Could you check a few things on this model? Use its own coordinates, in mm. A direction names the side the tool comes from. Coordinates: 2 decimals unless noted, no trailing zeros. Order: outer loops, then holes, each group sorted by start corner. A loop starts at its lowest first (then second) coordinate and runs counter-clockwise, first axis right, second up. Notation, with made-up numbers: (14, 76.5) -> (70, 76.5) arc R6 cw to (70, 80.5) -> close; hole circle Ø7 at (42.25, 82.25). An arc over 180 degrees is marked (long way). Put each result on its own line as item: value. Start each with the question number.
Q1. If we section it at C-C (z = 26): Please give me the cut outline in (x, y), and give its area (3 significant figures).
Q2. If we section it at B-B (y = -20): Please give me the cut outline in (x, z).
Q3. If we section it at D-D (y = -49): Please give me the cut outline in (x, z), and give its area (3 significant figures).
Q4. Please list where these lines run through material, in increasing order: line 1 along X through (y, z) = (-22.5, 0.75); line 2 along X through (y, z) = (-49, 41); line 3 along X through (y, z) = (-97, 1).
Q5. For faces 4 (the face through (24.73, -101.27, 1.38)), 5 (the face through (54.59, -59.16, 3.64)), which set-ups out of +Z, -Z, +X, -X, +Y, -Y let a thin tool reach every point of the face, with its end or its side?
Q6. We'd pull the mould along X, two halves only. Please class faces 1 (the face through (-46.17, -59.16, 3.6)), 2 (the face through (-48.21, -59.16, 1.68)), 3 (the face through (56.811, -12.675, 32.28)): +X half, -X half, draft (parallel to the pull), parting line (faces both ways), or undercut.
Q7. Will these pins go through, and if not, where does the flat tip stop? pin 1 (7 mm diameter, centred on x = -18.31, y = -22.5, fed in from +Z); pin 2 (4 mm diameter, centred on x = -4, y = -34.5, fed in from -Z); pin 3 (10 mm diameter, centred on x = 26.69, y = -22.5, fed in from +Z).
Q8. If we section it at A-A (z = 18): Please give me the cut outline in (x, y), and give its area (3 significant figures).
from build123d import *

# Parameters (mm, degrees)
F1_DEPTH = 120
F3_DEPTH = 3
F4_R     = 4.25
F5_DEPTH = 3


with BuildPart() as f1:
    # F0 (on Front) → F1 (new body)
    with BuildSketch(Plane.XZ):
        with BuildLine():
            ThreePointArc((-49.808191, 5.6), (-48.167989, 1.640202), (-44.208191, 0))
            Line((-44.208191, 0), (52.591809, 0))
            ThreePointArc((52.591809, 0), (56.551607, 1.640202), (58.191809, 5.6))
            Line((58.191809, 5.6), (58.191809, 52))
            Line((58.191809, 52), (55.391809, 52))
            Line((55.391809, 52), (55.391809, 5.6))
            ThreePointArc((55.391809, 5.6), (54.571708, 3.620101), (52.591809, 2.8))
            Line((52.591809, 2.8), (6.991809, 2.8))
            Line((6.991809, 2.8), (-44.208191, 2.8))
            ThreePointArc((-44.208191, 2.8), (-46.18809, 3.620101), (-47.008191, 5.6))
            Line((-47.008191, 5.6), (-47.008191, 52))
            Line((-47.008191, 52), (-49.808191, 52))
            Line((-49.808191, 52), (-49.808191, 5.6))
        make_face()
    extrude(amount=F1_DEPTH)

    # F2 (on face) → F3 (cut)
    with BuildSketch(Plane.YZ.offset(58.191809)):
        Polygon((-95, 52), (-120, 52), (-120, 12), align=None)
        with BuildLine():
            Line((-60, 64), (-60, 52))
            Line((-60, 52), (-60, 40))
            ThreePointArc((-60, 40), (-43.029437, 47.029437), (-36, 64))
            Line((-36, 64), (-60, 64))
        make_face()
        with BuildLine():
            Line((-60, 40), (-60, 52))
            Line((-60, 52), (-60, 64))
            Line((-60, 64), (-84, 64))
            ThreePointArc((-84, 64), (-76.970563, 47.029437), (-60, 40))
        make_face()
        with BuildLine():
            Line((-84, 64), (-60, 64))
            Line((-60, 64), (-36, 64))
            ThreePointArc((-36, 64), (-60, 88), (-84, 64))
        make_face()
        Polygon((0, 52), (-25, 52), (0, 12), align=None)
    extrude(amount=-F3_DEPTH, mode=Mode.SUBTRACT)

    # F4 (on face) → F5 (cut)
    with BuildSketch(Plane(origin=(0, 0, 0), x_dir=(1, 0, 0), z_dir=(0, 0, -1))):
        with BuildLine():
            Line((-22.558191, 97.5), (-18.308191, 97.5))
            Line((-18.308191, 97.5), (-14.058191, 97.5))
            ThreePointArc((-14.058191, 97.5), (-18.308191, 101.75), (-22.558191, 97.5))
        make_face()
        with BuildLine():
            Line((-18.308191, 93.25), (-18.308191, 97.5))
            Line((-18.308191, 97.5), (-22.558191, 97.5))
            ThreePointArc((-22.558191, 97.5), (-21.313395, 94.494796), (-18.308191, 93.25))
        make_face()
        with BuildLine():
            Line((-14.058191, 97.5), (-18.308191, 97.5))
            Line((-18.308191, 97.5), (-18.308191, 93.25))
            ThreePointArc((-18.308191, 93.25), (-15.302987, 94.494796), (-14.058191, 97.5))
        make_face()
        with BuildLine():
            ThreePointArc((30.941809, 97.5), (26.691809, 101.75), (22.441809, 97.5))
            Line((22.441809, 97.5), (30.941809, 97.5))
        make_face()
        with BuildLine():
            Line((30.941809, 97.5), (22.441809, 97.5))
            ThreePointArc((22.441809, 97.5), (26.691809, 93.25), (30.941809, 97.5))
        make_face()
        with BuildLine():
            ThreePointArc((-14.058191, 22.5), (-15.302987, 25.505204), (-18.308191, 26.75))
            ThreePointArc((-18.308191, 26.75), (-21.313395, 19.494796), (-14.058191, 22.5))
        make_face()
        with Locations((26.691809, 22.5)):
            Circle(F4_R)
    extrude(amount=-F5_DEPTH, mode=Mode.SUBTRACT)


solid = f1.part
The answers:
1. outline: (-49.81, -120) -> (-47.01, -120) -> (-47.01, 0) -> (-49.81, 0) -> close; (55.39, -111.25) -> (58.19, -111.25) -> (58.19, -8.75) -> (55.39, -8.75) -> close
1. area: 623 mm^2
2. outline: (-49.81, 5.6) arc R5.6 ccw to (-44.21, 0) -> (-21.75, 0) -> (-21.75, 2.8) -> (-44.21, 2.8) arc R2.8 cw to (-47.01, 5.6) -> (-47.01, 52) -> (-49.81, 52) -> close; (-14.87, 0) -> (23.25, 0) -> (23.25, 2.8) -> (-14.87, 2.8) -> close; (30.13, 0) -> (52.59, 0) arc R5.6 ccw to (58.19, 5.6) -> (58.19, 44) -> (55.39, 44) -> (55.39, 5.6) arc R2.8 cw to (52.59, 2.8) -> (30.13, 2.8) -> close
3. outline: (-49.81, 5.6) arc R5.6 ccw to (-44.21, 0) -> (52.59, 0) arc R5.6 ccw to (58.19, 5.6) -> (58.19, 42.67) -> (55.39, 42.67) -> (55.39, 5.6) arc R2.8 cw to (52.59, 2.8) -> (-44.21, 2.8) arc R2.8 cw to (-47.01, 5.6) -> (-47.01, 52) -> (-49.81, 52) -> close
3. area: 542 mm^2
4. line 1: -47.01 to -22.56, -14.06 to 22.44, 30.94 to 55.39
4. line 2: -49.81 to -47.01, 55.39 to 58.19
4. line 3: -47.4 to -22.53, -14.09 to 22.47, 30.91 to 55.79
5. face 4: +Z, -Z
5. face 5: +Z, +Y, -Y
6. face 1: undercut
6. face 2: -X half
6. face 3: draft
7. pin 1: through
7. pin 2: z = 0
7. pin 3: z = 2.8
8. outline: (-49.81, -120) -> (-47.01, -120) -> (-47.01, 0) -> (-49.81, 0) -> close; (55.39, -116.25) -> (58.19, -116.25) -> (58.19, -3.75) -> (55.39, -3.75) -> close
8. area: 651 mm^2
